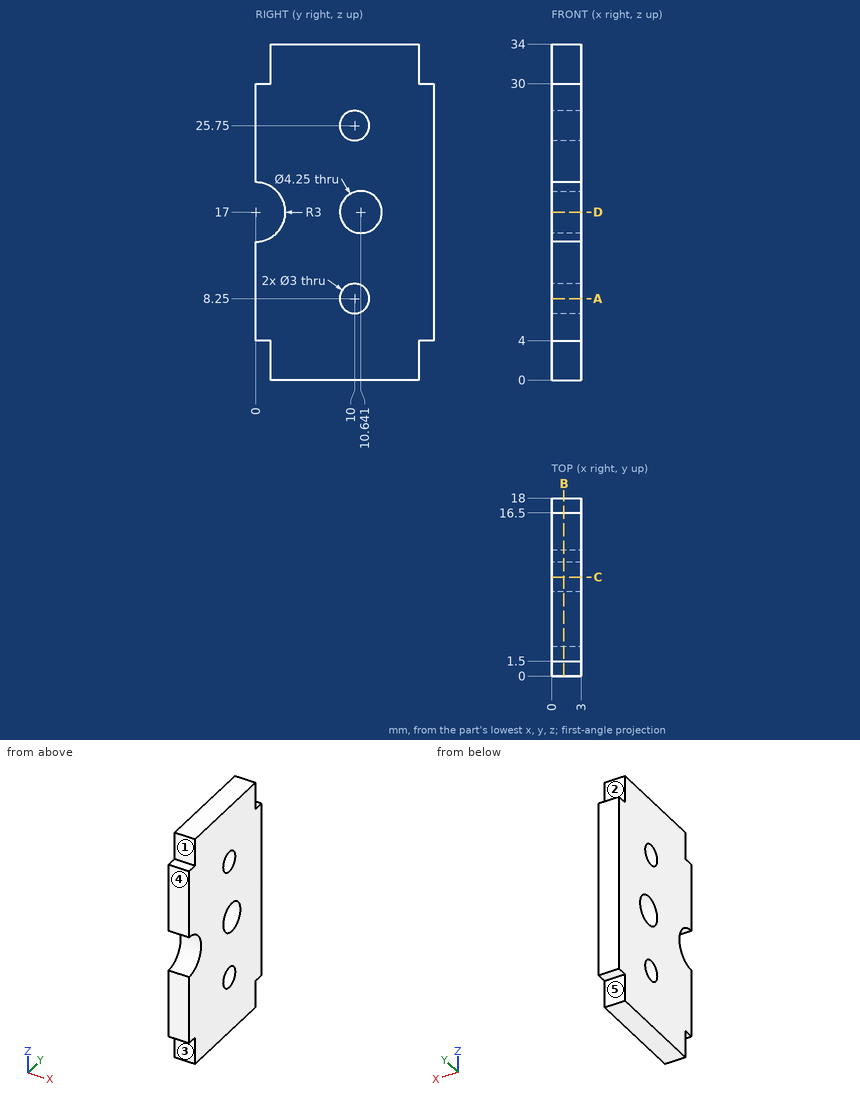
For this review, use the dimensioned drawing (mm, ordinates from the lowest corner) and the shaded views. A direction names the side the tool comes from. Give positions to 0.01 mm unless a question says otherwise; leave off trailing zeros. Loops run counter-clockwise (first coordinate to the right, second up) from the corner with the lowest first, then second, coordinate; pieces in that order, holes last. Notation, with made-up numbers: (61, 66) -> (77, 66) arc R22 cw to (77, 93) -> close; hole circle Ø2 at (-14.5, -22). An arc over 180 degrees is marked (long way). Use CSV: the item, a comma, the result in double quotes.
1. Consider section A-A, the plane z = 8.25. Write out the cut boundary in (x, y).
Result:
outline,"(0, 0) -> (3, 0) -> (3, 8.5) -> (0, 8.5) -> close; (0, 11.5) -> (3, 11.5) -> (3, 18) -> (0, 18) -> close"
2. Consider section C-C, the plane y = 10. Write out the cut boundary in (x, z).
Result:
outline,"(0, 0) -> (3, 0) -> (3, 6.75) -> (0, 6.75) -> close; (0, 9.75) -> (3, 9.75) -> (3, 14.97) -> (0, 14.97) -> close; (0, 19.03) -> (3, 19.03) -> (3, 24.25) -> (0, 24.25) -> close; (0, 27.25) -> (3, 27.25) -> (3, 34) -> (0, 34) -> close"
3. Machinability: for the marked faces 1, 2, 3, 4 and 5, which of the approach directions +Z, -Z, +X, -X, +Y, -Y give a long, thin tool a straight path to every point of the face, cutting with its end or side? Answer none if there is none.
Result:
face 1,"+Z, +X, -X, -Y"
face 2,"+Z, +X, -X, +Y"
face 3,"-Z, +X, -X, -Y"
face 4,"+Z, -Z, +X, -X, -Y"
face 5,"-Z, +X, -X, +Y"
4. For P1, Ø1.5, axis at x = 2, z = 17, coming from the -Y side; P2, Ø1.5, axis at x = 1.5, z = 1.5, coming from the -Y side; P3, Ø0.8, axis at x = 2, y = 17.5, coming from the -Z side; P4, Ø6, axis at y = 10, z = 8.5, coming from the +X side, all flat-tipped, find the tip position at first contact; note any pin that passes through.
Result:
P1,"stops at y = 2.9"
P2,"stops at y = 1.5"
P3,"stops at z = 4"
P4,"stops at x = 3"
5. Consider section B-B, the plane x = 1.25. Write out the cut boundary in (y, z) (3 decimals).
Result:
outline,"(0, 4) -> (1.5, 4) -> (1.5, 0) -> (16.5, 0) -> (16.5, 4) -> (18, 4) -> (18, 30) -> (16.5, 30) -> (16.5, 34) -> (1.5, 34) -> (1.5, 30) -> (0, 30) -> (0, 20) arc R3 cw to (0, 14) -> close; hole circle Ø3 at (10, 8.25); hole circle Ø3 at (10, 25.75); hole circle Ø4.25 at (10.641, 17)"
6. Consider section D-D, the plane z = 17. Write out the cut boundary in (x, y).
Result:
outline,"(0, 3) -> (3, 3) -> (3, 8.52) -> (0, 8.52) -> close; (0, 12.77) -> (3, 12.77) -> (3, 18) -> (0, 18) -> close"
7. To check wall thickness, follow probe 1 along Y at (x, z) = (2.3, 17); probe 2 along Y at (x, z) = (2.1, 25.75); probe 3 along Z at (x, y) = (2.25, 11.25) (1 decimal). State the ranges of each line that lie inside material, in increasing order. Write a range as from..to.
Result:
probe 1,"y = 3..8.52, 12.77..18"
probe 2,"y = 0..8.5, 11.5..18"
probe 3,"z = 0..7.4, 9.1..15, 19..24.9, 26.6..34"
